from build123d import *

# Parameters (mm, degrees)
SKETCH_1_R               = 30
EXTRUDE_1_DEPTH          = 6
SKETCH_2_R               = 6
EXTRUDE_2_DEPTH          = 3
SKETCH_3_R               = 5
EXTRUDE_3_DEPTH          = 24
CUT_EXTRUDE_START        = -12
SKETCH_4_OUTSIDE_W       = 80.208
SKETCH_4_OUTSIDE_H       = 80.208
SKETCH_4_OUTSIDE_R       = 4.75
CUT_EXTRUDE_1_DEPTH      = 1.1
SKETCH_5_R               = 2.6
CUT_EXTRUDE_2_DEPTH      = 51.289163843
CHAMFER_1_SIZE           = 3
CHAMFER_2_SIZE           = 0.5
SKETCH_6_R               = 13
CUT_EXTRUDE_3_DEPTH      = 1.2
PATTERN_CIRCULAR_1_COUNT = 6


with BuildPart() as part:
    # 草图1 → 凸台-拉伸1 (new body)
    with BuildSketch(Plane(origin=(0, 0, 0), x_dir=(1, 0, 0), z_dir=(0, 1, 0))):
        with Locations(Location((0, 0, 0), (0, 0, 270))):
            Circle(SKETCH_1_R)
    extrude(amount=EXTRUDE_1_DEPTH)

    # 草图2 → 凸台-拉伸2 (add)
    with BuildSketch(Plane(origin=(0, 6, 0), x_dir=(1, 0, 0), z_dir=(0, 1, 0))):
        with Locations(Location((0, 0, 0), (0, 0, 270))):
            Circle(SKETCH_2_R)
    extrude(amount=EXTRUDE_2_DEPTH)

    # 草图3 → 凸台-拉伸3 (add)
    with BuildSketch(Plane(origin=(0, 9, 0), x_dir=(1, 0, 0), z_dir=(0, 1, 0))):
        with Locations(Location((0, 0, 0), (0, 0, 270))):
            Circle(SKETCH_3_R)
    extrude(amount=EXTRUDE_3_DEPTH)

    # 草图4 outside → 切除-拉伸1 (cut)
    with BuildSketch(Plane(origin=(0, 33, 0), x_dir=(1, 0, 0), z_dir=(0, 1, 0)).offset(CUT_EXTRUDE_START)):
        Rectangle(SKETCH_4_OUTSIDE_W, SKETCH_4_OUTSIDE_H)
        with Locations(Location((0, 0, 0), (0, 0, 270))):
            Circle(SKETCH_4_OUTSIDE_R, mode=Mode.SUBTRACT)
    extrude(amount=CUT_EXTRUDE_1_DEPTH, mode=Mode.SUBTRACT)

    # 草图5 → 切除-拉伸2 (cut, through all)
    with BuildSketch(Plane(origin=(0, 6, 0), x_dir=(1, 0, 0), z_dir=(0, 1, 0))):
        with Locations(Location((0, 23, 0), (0, 0, 270))):
            Circle(SKETCH_5_R)
        with Locations(Location((19.918584287, 11.5, 0), (0, 0, 270))):
            Circle(SKETCH_5_R)
        with Locations(Location((19.918584287, -11.5, 0), (0, 0, 270))):
            Circle(SKETCH_5_R)
        with Locations(Location((0, -23, 0), (0, 0, 270))):
            Circle(SKETCH_5_R)
        with Locations(Location((-19.918584287, -11.5, 0), (0, 0, 270))):
            Circle(SKETCH_5_R)
        with Locations(Location((-19.918584287, 11.5, 0), (0, 0, 270))):
            Circle(SKETCH_5_R)
    extrude(amount=-CUT_EXTRUDE_2_DEPTH, mode=Mode.SUBTRACT)

    # 倒角1
    chamfer_1_edges = [part.edges().sort_by_distance(p)[0] for p in [
        (0, 6, -6),
    ]]
    chamfer(chamfer_1_edges, length=CHAMFER_1_SIZE - 0.0001)  # a hair under: the kernel refuses the full size

    # 倒角2
    chamfer_2_edges = [part.edges().sort_by_distance(p)[0] for p in [
        (0, 33, -5),
    ]]
    chamfer(chamfer_2_edges, length=CHAMFER_2_SIZE)

    # 草图6 → 切除-拉伸3 (cut)
    with BuildSketch(Plane.XZ):
        with Locations(Location((0, 0, 0), (0, 0, 270))):
            Circle(SKETCH_6_R)
    extrude(amount=-CUT_EXTRUDE_3_DEPTH, mode=Mode.SUBTRACT)

    # 草图7 → 切除-旋转1 (revolve, cut)
    with BuildSketch(Plane(origin=(0, 0, 0), x_dir=(0, 0, -1), z_dir=(1, 0, 0))):
        Polygon((-28, 6), (-23, 6), (-23, 1.9), (-23.9, 1.9), align=None)
    cut_revolve_1 = revolve(axis=Axis((0, 6, 23), (0, -1, 0)), mode=Mode.SUBTRACT)

    # 阵列(圆周)1: 切除-旋转1 ×6 about axis
    pattern_circular_1_axis = Axis((0, 0, 0), (0, 1, 0))
    for i in range(1, PATTERN_CIRCULAR_1_COUNT):
        add(cut_revolve_1.rotate(pattern_circular_1_axis, i * 360 / PATTERN_CIRCULAR_1_COUNT), mode=Mode.SUBTRACT)


solid = part.part
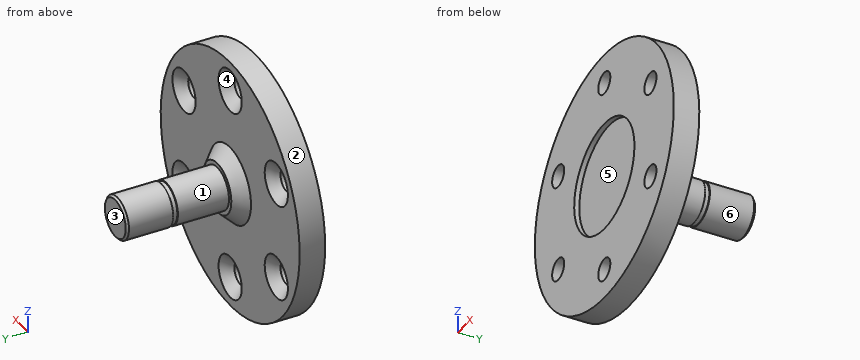
Can you work these out from the model? Positions are in its coordinate system, mm. Face numbers are marked on the shaded views. A direction names the side the tool comes from. Round coordinates to 2 decimals unless told otherwise and drop trailing zeros. Write each loop counter-clockwise with the first axis right and the second up, starting at its lowest first coordinate (ties: lowest second). Pieces come first, ordered by that corner, then holes. Notation, with made-up numbers: (-27, -19) - (-23, -19) arc R16 ccw to (-23, 9) - close; hole circle Ø2 at (-3, 6). An arc over 180 degrees is marked (long way). Write each question's results on one line, items separated by ' | '. Start each with the question number.
1) We'd pull the mould along Z, two halves only. Please class the marked faces 3, 4, 5 and 6: released by +Z, released by -Z, zero draft, split by the parting line, or undercut.
2) Suppose I cut it at D-D (y = 27.5). List the corners of the cut face in (x, z) for me.
3) Suppose I cut it at B-B (x = 0). Give the number of separate pieces and of enclosed holes in the cut face, and give its area (3 significant figures).
4) Please list where these lines run through material, in increasing order: line 1 (X direction, y = 2.3, z = -11.5); line 2 (Y direction, x = 8, z = -23); line 3 (Y direction, x = -2, z = -4.5).
5) Suppose I cut it at C-C (z = -23). List the corners of the cut face in (x, y) for me.
6) Which directions (+Z, -Z, +X, -X, +Y, -Y) give clear straight access to the entire face, cutting with the end or side of a thin tool? Please do the marked faces 1 and 2.
7) For pin 1 Ø6 at (x, z) = (-19.92, 11.5) entering from +Y; pin 2 Ø10 at (x, z) = (16, 10) entering from +Y; pin 3 Ø8 at (x, y) = (-4.5, 9.5) entering from -Z, each with a flat end and sliding along its axis, tell me the tip position at first contact or that it passes through.
Here are the results:
1) face 3: zero draft | face 4: undercut | face 5: undercut | face 6: split by the parting line
2) outline: circle Ø10 at (0, 0)
3) separate pieces: 3 | enclosed holes: 0 | area: 539 mm2
4) line 1: x = -27.71 to -22.52, -17.32 to 17.32, 22.52 to 27.71 | line 2: y = 0 to 6 | line 3: y = 1.2 to 21, 22.1 to 32.58
5) outline: (-19.26, 0) - (-2.6, 0) - (-2.6, 3.6) - (-5, 6) - (-19.26, 6) - close; (2.6, 0) - (19.26, 0) - (19.26, 6) - (5, 6) - (2.6, 3.6) - close
6) face 1: +Y | face 2: +Y, -Y
7) pin 1: stops at y = 4 | pin 2: stops at y = 6 | pin 3: stops at z = -29.89
